Design review of the part built by this model. Coordinates are the model's own, in mm. A direction names the side the tool comes from. Coordinates: 2 decimals unless noted, no trailing zeros. Loops run counter-clockwise (first coordinate to the right, second up) from the corner with the lowest first, then second, coordinate; pieces in that order, holes last. Notation, with made-up numbers: (54.25, 72.25) -> (87.25, 72.25) arc R28 ccw to (87.25, 105.25) -> close; hole circle Ø1 at (-31, -9). An arc over 180 degrees is marked (long way). Answer in a Markdown table with one row per item.
```python
from build123d import *

# Parameters (mm, degrees)
SKETCH_1_R      = 10.175
SKETCH_1_R_2    = 1.375
SKETCH_1_R_3    = 0.7
EXTRUDE_1_DEPTH = 2.2
SKETCH_2_R      = 4.85
SKETCH_2_R_2    = 3
EXTRUDE_2_DEPTH = 4.5


with BuildPart() as part:
    # 草圖1 → 填料-伸長1 (new body)
    with BuildSketch(Plane.XY):
        Circle(SKETCH_1_R)
        Circle(SKETCH_1_R_2, mode=Mode.SUBTRACT)
        with Locations((7.925, 0)):
            Circle(SKETCH_1_R_3, mode=Mode.SUBTRACT)
        with Locations((7.925, 3.4)):
            Circle(SKETCH_1_R_3, mode=Mode.SUBTRACT)
        with Locations((7.925, -3.4)):
            Circle(SKETCH_1_R_3, mode=Mode.SUBTRACT)
        with Locations((-7.925, 0)):
            Circle(SKETCH_1_R_3, mode=Mode.SUBTRACT)
        with Locations((-7.925, 3.4)):
            Circle(SKETCH_1_R_3, mode=Mode.SUBTRACT)
        with Locations((-7.925, -3.4)):
            Circle(SKETCH_1_R_3, mode=Mode.SUBTRACT)
        with Locations((0, -7.925)):
            Circle(SKETCH_1_R_3, mode=Mode.SUBTRACT)
        with Locations((-3.4, -7.925)):
            Circle(SKETCH_1_R_3, mode=Mode.SUBTRACT)
        with Locations((3.4, -7.925)):
            Circle(SKETCH_1_R_3, mode=Mode.SUBTRACT)
        with Locations((0, 7.925)):
            Circle(SKETCH_1_R_3, mode=Mode.SUBTRACT)
        with Locations((3.4, 7.925)):
            Circle(SKETCH_1_R_3, mode=Mode.SUBTRACT)
        with Locations((-3.4, 7.925)):
            Circle(SKETCH_1_R_3, mode=Mode.SUBTRACT)
    extrude(amount=EXTRUDE_1_DEPTH)

    # 草圖2 → 填料-伸長2 (add)
    with BuildSketch(Plane.XY.offset(2.2)):
        Circle(SKETCH_2_R)
        Circle(SKETCH_2_R_2, mode=Mode.SUBTRACT)
    extrude(amount=EXTRUDE_2_DEPTH)


solid = part.part
```
(1) Tool access review of faces 1 (the cylindrical face through (-8.624, 0.031, 1.085)), 2 (the cylindrical face through (-3, 0, 4)): name each direction out of +Z, -Z, +X, -X, +Y, -Y from which nothing blocks a thin tool from reaching the whole face with its end or side.
Evaluation:
| item | result |
|---|---|
| face 1 | +Z, -Z |
| face 2 | +Z |
(2) Take a section at A-A on y = 0. Give the boundary of the cut face in (x, z) (3 decimals), and give its area (3 significant figures).
Evaluation:
| item | result |
|---|---|
| outline | (-10.175, 0) -> (-8.625, 0) -> (-8.625, 2.2) -> (-10.175, 2.2) -> close; (-7.225, 0) -> (-1.375, 0) -> (-1.375, 2.2) -> (-3, 2.2) -> (-3, 6.7) -> (-4.85, 6.7) -> (-4.85, 2.2) -> (-7.225, 2.2) -> close; (1.375, 0) -> (7.225, 0) -> (7.225, 2.2) -> (4.85, 2.2) -> (4.85, 6.7) -> (3, 6.7) -> (3, 2.2) -> (1.375, 2.2) -> close; (8.625, 0) -> (10.175, 0) -> (10.175, 2.2) -> (8.625, 2.2) -> close |
| area | 49.2 mm² |
(3) To check wall thickness, follow probe 1 along Y at (x, z) = (8, 0.5); probe 2 along X at (y, z) = (8.5, 1.75); probe 3 along Z at (x, y) = (-1, -6.25). State the ranges of each line that lie inside material, in increasing order.
Evaluation:
| item | result |
|---|---|
| probe 1 | y = -6.29 to -4.1, -2.7 to -0.7, 0.7 to 2.7, 4.1 to 6.29 |
| probe 2 | x = -5.59 to -3.8, -3 to -0.4, 0.4 to 3, 3.8 to 5.59 |
| probe 3 | z = 0 to 2.2 |
(4) Take a section at C-C on y = -3.4. Give the boundary of the cut face in (x, z) (3 decimals).
Evaluation:
| item | result |
|---|---|
| outline | (-9.59, 0) -> (-8.625, 0) -> (-8.625, 2.2) -> (-9.59, 2.2) -> close; (-7.225, 0) -> (7.225, 0) -> (7.225, 2.2) -> (3.459, 2.2) -> (3.459, 6.7) -> (-3.459, 6.7) -> (-3.459, 2.2) -> (-7.225, 2.2) -> close; (8.625, 0) -> (9.59, 0) -> (9.59, 2.2) -> (8.625, 2.2) -> close |
(5) For pin 1 (2 mm diameter, centred on x = 0, y = -7.925, fed in from -Z); pin 2 (1.6 mm diameter, centred on x = 7.925, y = 0, fed in from +Z); pin 3 (2 mm diameter, centred on x = -4, z = 1, fed in from +Y); pin 4 (1.5 mm diameter, centred on x = 5.5, z = 2, fed in from +Y), all flat-tipped, find the tip position at first contact; note any pin that passes through.
Evaluation:
| item | result |
|---|---|
| pin 1 | stops at z = 0 |
| pin 2 | stops at z = 2.2 |
| pin 3 | stops at y = 9.72 |
| pin 4 | stops at y = 9 |
(6) Draft analysis for pull direction Y (two halves, no side actions). For faces 3 (the cylindrical face through (-2.206, -9.933, 1.085)), 4 (the flat face through (-2.4, -4.4, 2.2)), 5 (the cylindrical face through (-0.3, -1.34, 1.08)), state which applies: pulls with the +Y half, pulls with the -Y half, needs draft (parallel to the pull), parting line crosses it, or undercut.
Evaluation:
| item | result |
|---|---|
| face 3 | parting line crosses it |
| face 4 | needs draft |
| face 5 | undercut |
